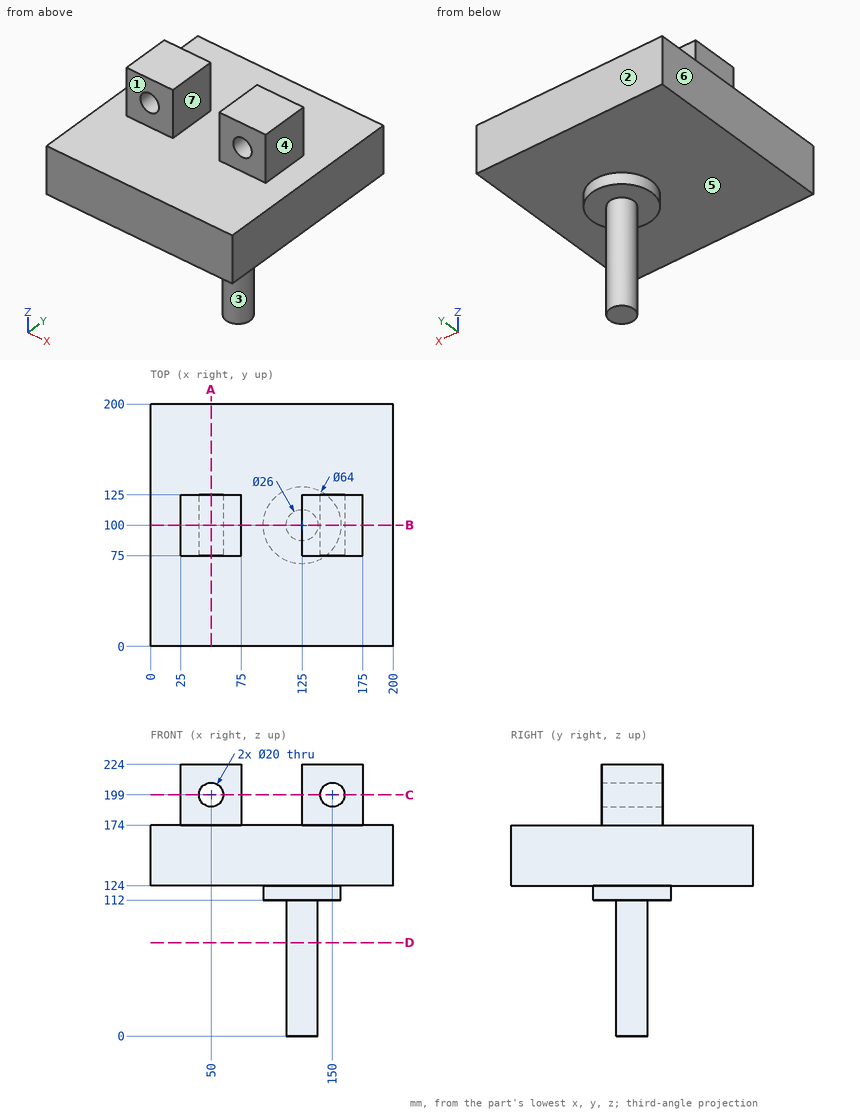
Geometry: see drawing. Coordinates: mm, zero at the bounding-box minimum. A direction names the side the tool comes from. Give positions to 0.01 mm unless a question says otherwise; leave off trailing zeros. Order: outer loops, then holes, each group sorted by start corner. A loop starts at its lowest first (then second) coordinate and runs counter-clockwise, first axis right, second up. Notation, with made-up numbers: (22, -35.75) - (65, -35.75) arc R10 cw to (65, -28.75) - close; hole circle Ø5 at (52.25, 45). An arc over 180 degrees is marked (long way). Use a Markdown table: item, result.
(1) Section query C-C (z = 199). Output: boundary loops of the cut face in (x, y).
Computed values:
| item | result |
|---|---|
| outline | (25, 75) - (40, 75) - (40, 125) - (25, 125) - close; (60, 75) - (75, 75) - (75, 125) - (60, 125) - close; (125, 75) - (140, 75) - (140, 125) - (125, 125) - close; (160, 75) - (175, 75) - (175, 125) - (160, 125) - close |
(2) Section query B-B (y = 100). Output: boundary loops of the cut face in (x, z).
Computed values:
| item | result |
|---|---|
| outline | (0, 124) - (93, 124) - (93, 112) - (112, 112) - (112, 0) - (138, 0) - (138, 112) - (157, 112) - (157, 124) - (200, 124) - (200, 174) - (175, 174) - (175, 224) - (125, 224) - (125, 174) - (75, 174) - (75, 224) - (25, 224) - (25, 174) - (0, 174) - close; hole circle Ø20 at (50, 199); hole circle Ø20 at (150, 199) |
(3) Section query A-A (x = 50). Output: boundary loops of the cut face in (y, z).
Computed values:
| item | result |
|---|---|
| outline | (0, 124) - (200, 124) - (200, 174) - (125, 174) - (125, 189) - (75, 189) - (75, 174) - (0, 174) - close; (75, 209) - (125, 209) - (125, 224) - (75, 224) - close |
(4) Access query for the marked faces 1, 2, 3 and 4. Directions: +Z, -Z, +X, -X, +Y, -Y. A direction counts if a zero-diameter tool reaches every point of the face in a straight line with its end or side. Return the directions, or none.
Computed values:
| item | result |
|---|---|
| face 1 | +Z, +X, -X, -Y |
| face 2 | +Z, -Z, +X, -X, +Y |
| face 3 | -Z |
| face 4 | +Z, +X, +Y, -Y |
(5) Section query D-D (z = 77). Output: boundary loops of the cut face in (x, y).
Computed values:
| item | result |
|---|---|
| outline | circle Ø26 at (125, 100) |
(6) Draft query along X for the marked faces 5, 6 and 7. Return one class per face: released by +X, released by -X, zero draft, split by the parting line, or undercut.
Computed values:
| item | result |
|---|---|
| face 5 | zero draft |
| face 6 | released by -X |
| face 7 | undercut |
(7) Pin query (flat end, axial travel): pin 1 (6 mm diameter, centred on x = 121, z = 55.5, fed in from -Y); pin 2 (10 mm diameter, centred on y = 100.5, z = 109, fed in from -X); pin 3 (1.5 mm diameter, centred on x = 78.5, y = 85.5, fed in from -Z). Return the tip coordinate at first contact, or that it passes through.
Computed values:
| item | result |
|---|---|
| pin 1 | stops at y = 87.04 |
| pin 2 | stops at x = 93 |
| pin 3 | stops at z = 124 |
(8) Line query: line 1 (X direction, y = 114, z = 199); line 2 (Z direction, x = 150, y = 95.5); line 3 (Z direction, x = 50, y = 113). Output: solid intervals per line, ascending. Write a range as from..to.
Computed values:
| item | result |
|---|---|
| line 1 | x = 25..40, 60..75, 125..140, 160..175 |
| line 2 | z = 112..189, 209..224 |
| line 3 | z = 124..189, 209..224 |
